Build history of the part. All positions in model axes, mm. Face numbers are marked on the shaded views. Give positions to 0.01 mm unless a question says otherwise; leave off trailing zeros. Loops run counter-clockwise (first coordinate to the right, second up) from the corner with the lowest first, then second, coordinate; pieces in that order, holes last. Notation, with made-up numbers: (70, 88) -> (81, 88) arc R13 ccw to (81, 112) -> close; hole circle Ø9 at (6.5, 35.5). An arc over 180 degrees is marked (long way). One line per question, with ' | ' between items. Start each with the question number.
(1) Flat gauge pins, fed straight in: pin 1 Ø4 at (y, z) = (5.5, -2.5) entering from +X; pin 2 Ø4.5 at (x, z) = (0, 0) entering from -Y. Where does each tip first touch, or does it go through?
(2) Slice it at A-A, the plane x = 0. Write the cut outline in (y, z) (3 decimals), then the cut area to 3 significant figures.
(3) Slice it at C-C, the plane z = 0.25. Write the cut outline in (x, y), then the cut area to 3 significant figures.
(4) Slice it at D-D, the plane x = 4.25. Write the cut outline in (y, z).
(5) Slice it at B-B, the plane y = 14. Write the cut outline in (x, z) (3 decimals), then the cut area to 3 significant figures.
(6) Drill centre lines: L1, parallel to Z at x = 0, y = 4 (3 decimals); L2, parallel to X at y = 2.5, z = 1.5; L3, parallel to Z at x = 1.25, y = 14 (3 decimals). Where is each one in solid material? Low to high. Write a range as from..to.
(7) Mould opens along X. For the marked faces 1, 2, 3 and 4 say: pulls with the +X half, pulls with the -X half, needs draft (parallel to the pull), parting line crosses it, or undercut.
```python
from build123d import *

# Parameters (mm, degrees)
BOSS_EXTRUDE1_DEPTH    = 18.67
F_10_24_TAPPED_HOLE1_D = 4.826


with BuildPart() as part:
    # Sketch1 → Boss-Extrude1 (new body)
    with BuildSketch(Plane(origin=(0, 0, 0), x_dir=(1, 0, 0), z_dir=(0, 1, 0))):
        Polygon((4.58993464, 0), (2.29496732, 3.975), (-2.29496732, 3.975), (-4.58993464, 0), (-2.29496732, -3.975), (2.29496732, -3.975), align=None)
    extrude(amount=BOSS_EXTRUDE1_DEPTH)

    # #10-24 Tapped Hole1 (through all)
    with Locations(Plane(origin=(0, 18.67, 0), x_dir=(-1, 0, 0), z_dir=(0, 1, 0))):
        with Locations((0, 0)):
            Hole(F_10_24_TAPPED_HOLE1_D / 2)


solid = part.part
```
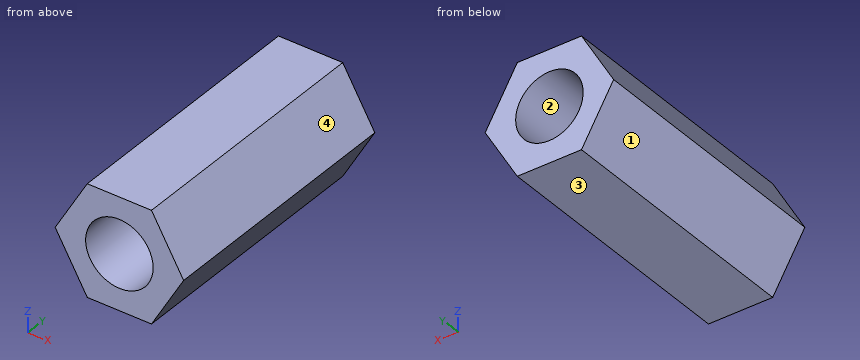
Final values:
1) pin 1: x = 4.3 | pin 2: through
2) outline: (0, -3.975) -> (18.67, -3.975) -> (18.67, -2.413) -> (0, -2.413) -> close; (0, 2.413) -> (18.67, 2.413) -> (18.67, 3.975) -> (0, 3.975) -> close | area: 58.3 mm2
3) outline: (-4.45, 0) -> (-2.4, 0) -> (-2.4, 18.67) -> (-4.45, 18.67) -> close; (2.4, 0) -> (4.45, 0) -> (4.45, 18.67) -> (2.4, 18.67) -> close | area: 76.4 mm2
4) outline: (0, -0.59) -> (18.67, -0.59) -> (18.67, 0.59) -> (0, 0.59) -> close
5) outline: (-4.59, 0) -> (-2.295, -3.975) -> (2.295, -3.975) -> (4.59, 0) -> (2.295, 3.975) -> (-2.295, 3.975) -> close; hole circle Ø4.826 at (0, 0) | area: 36.4 mm2
6) L1: -3.975..-2.413, 2.413..3.975 | L2: -3.72..-1.89, 1.89..3.72 | L3: -3.975..-2.064, 2.064..3.975
7) face 1: pulls with the -X half | face 2: undercut | face 3: needs draft | face 4: pulls with the +X half
